Verification items for the finished model (mm, model axes). A direction names the side the tool comes from. Round coordinates to 2 decimals unless told otherwise and drop trailing zeros. Order: outer loops, then holes, each group sorted by start corner. A loop starts at its lowest first (then second) coordinate and runs counter-clockwise, first axis right, second up. Notation, with made-up numbers: M -15.5,8 L 5.5,8 A24 ccw 5.5,31 Z; hole C -9,43 d11. An arc over 180 degrees is marked long. Use one line per item in the form item = value. Start each with the question number.
Item 1: Release check for a two-part mould opening along X. For faces 1 (the flat face through (-39, 5, -6)), 2 (the flat face through (-1, 7, -10)) record: +X half, -X half, draft (parallel to the pull), parting line (faces both ways), or undercut.
Item 2: Cross-section at B-B on x = -41. Enter the section's corners in (y, z), then the cut area to 3 significant figures.
Item 3: Tool access check on faces 3 (the cylindrical face through (-44.173, 1.972, 2.205)), 4 (the flat face through (-21, 4.5, 6)), 5 (the cylindrical face through (-39.61, 6.03, 2.39)). Record the directions out of +Z, -Z, +X, -X, +Y, -Y that give a thin tool (end or side, any length) a straight path to the whole face; none if there is none.
Item 4: Cross-section at C-C on y = 7.25. Enter the section's corners in (x, z), then the cut area to 3 significant figures.
Item 5: Thickness scan on probe 1 along X at (y, z) = (2.5, 1.5); probe 2 along X at (y, z) = (6.25, 4.25); probe 3 along Z at (x, y) = (-31, 7.5). Record the ranges inside material, lowest first. Write a range as [from, to].
Item 6: Cross-section at A-A on z = 6. Enter the section's corners in (x, y), then the cut area to 3 significant figures.
Item 7: Go/stop test with flat-tipped pins: pin 1 Ø5 at (x, z) = (41, 2) entering from -Y; pin 2 Ø1.5 at (x, z) = (-15.5, 4.5) entering from +Y; pin 3 Ø4 at (x, z) = (14, 5) entering from +Y. Record where each tip stops, or that it passes through.
Item 8: Cross-section at D-D on x = 32. Enter the section's corners in (y, z), then the cut area to 3 significant figures.
from build123d import *

# Parameters (mm, degrees)
ESQUISSE1_W             = 90
ESQUISSE1_H             = 25
BOSS_EXTRU_1_DEPTH      = 8
ESQUISSE3_R             = 1.65
ENL_V_MAT_EXTRU_1_DEPTH = 48.384069053
ESQUISSE4_R             = 3.25
ENL_V_MAT_EXTRU_2_DEPTH = 4
EMPREINTE1_START        = -10
EMPREINTE1_DEPTH        = 8
EMPREINTE1_START_2      = 2
EMPREINTE1_2_DEPTH      = 8
EMPREINTE1_START_3      = -38.94589
EMPREINTE1_3_DEPTH      = 77.9
EMPREINTE1_START_4      = -41
EMPREINTE1_4_DEPTH      = 82


with BuildPart() as part:
    # Esquisse1 → Boss.-Extru.1 (new body)
    with BuildSketch(Plane(origin=(0, 0, 0), x_dir=(1, 0, 0), z_dir=(0, 1, 0))):
        Rectangle(ESQUISSE1_W, ESQUISSE1_H)
    extrude(amount=BOSS_EXTRU_1_DEPTH)

    # Esquisse3 → Enlèv. mat.-Extru.1 (cut, through all)
    with BuildSketch(Plane(origin=(0, 8, 0), x_dir=(1, 0, 0), z_dir=(0, 1, 0))):
        with Locations(Location((0, -6, 0), (0, 0, 270))):
            Circle(ESQUISSE3_R)
        with Locations(Location((41, -1.5, 0), (0, 0, 270))):
            Circle(ESQUISSE3_R)
        with Locations(Location((-41, -1.5, 0), (0, 0, 270))):
            Circle(ESQUISSE3_R)
    extrude(amount=-ENL_V_MAT_EXTRU_1_DEPTH, mode=Mode.SUBTRACT)

    # Esquisse4 → Enlèv. mat.-Extru.2 (cut)
    with BuildSketch(Plane.XZ):
        with Locations(Location((-41, 1.5, 0), (0, 0, 270))):
            Circle(ESQUISSE4_R)
        with Locations(Location((41, 1.5, 0), (0, 0, 270))):
            Circle(ESQUISSE4_R)
        with Locations(Location((0, 6, 0), (0, 0, 270))):
            Circle(ESQUISSE4_R)
    extrude(amount=-ENL_V_MAT_EXTRU_2_DEPTH, mode=Mode.SUBTRACT)

    # Empreinte1: read off the stored shape, not the designer's step
    # Empreinte1 outline → Empreinte1 (cut)
    with BuildSketch(Plane.XY.offset(EMPREINTE1_START)):
        Polygon((40, 8), (-40, 8), (-40, 6), (-38.5, 4.5), (38.5, 4.5), (40, 6), align=None)
    extrude(amount=EMPREINTE1_DEPTH, mode=Mode.SUBTRACT)

    # Empreinte1 2 outline → Empreinte1 2 (cut)
    with BuildSketch(Plane.XY.offset(EMPREINTE1_START_2)):
        Polygon((6.5, 4.5), (22.5, 4.5), (24, 6), (24, 8), (5, 8), (5, 6), align=None)
        Polygon((-35.5, 4.5), (-6.5, 4.5), (-5, 6), (-5, 8), (-37, 8), (-37, 6), align=None)
    extrude(amount=EMPREINTE1_2_DEPTH, mode=Mode.SUBTRACT)

    # Empreinte1 3 outline → Empreinte1 3 (add)
    with BuildSketch(Plane.YZ.offset(EMPREINTE1_START_3)):
        Polygon((4.5, 2), (6, 2), (4.5, 3.5), align=None)
        Polygon((4.5, 10), (4.5, 8.5), (6, 10), align=None)
        Polygon((6, -10), (4.5, -8.5), (4.5, -10), align=None)
        Polygon((4.5, -2), (4.5, -3.5), (6, -2), align=None)
    extrude(amount=EMPREINTE1_3_DEPTH)

    # Empreinte1 4 outline → Empreinte1 4 (add)
    with BuildSketch(Plane.YZ.offset(EMPREINTE1_START_4)):
        Polygon((6, -10), (4.5, -8.5), (4.5, -10), align=None)
        Polygon((4.5, -2), (4.5, -3.5), (6, -2), align=None)
    extrude(amount=EMPREINTE1_4_DEPTH)


solid = part.part
Output values:
q1.face_1 = undercut
q1.face_2 = undercut
q2.outline = M 0,-12.5 L 8,-12.5 L 8,-0.15 L 4,-0.15 L 4,-1.75 L 0,-1.75 Z; M 0,4.75 L 4,4.75 L 4,3.15 L 8,3.15 L 8,12.5 L 0,12.5 Z
q2.area = 161 mm2
q3.face_3 = -Y
q3.face_4 = +Y
q3.face_5 = +Y, -Y
q4.outline = M -45,-12.5 L 45,-12.5 L 45,12.5 L -45,12.5 Z; hole C -41,1.5 d3.3; hole M -40,-10 L 40,-10 L 40,-2 L -40,-2 Z; hole M -37,2 L -5,2 L -5,10 L -37,10 Z; hole C 0,6 d3.3; hole M 5,2 L 24,2 L 24,10 L 5,10 Z; hole C 41,1.5 d3.3
q4.area = 1,180 mm2
q5.probe_1 = [-45, -44.25], [-37.75, 37.75], [44.25, 45]
q5.probe_2 = [-45, -37], [-5, 5], [24, 45]
q5.probe_3 = [-12.5, -10], [-2, 2], [10, 12.5]
q6.outline = M -45,0 L -3.25,0 L -3.25,4 L -1.65,4 L -1.65,8 L -5,8 L -5,6 L -6.5,4.5 L -35.5,4.5 L -37,6 L -37,8 L -45,8 Z; M 1.65,4 L 3.25,4 L 3.25,0 L 45,0 L 45,8 L 24,8 L 24,6 L 22.5,4.5 L 6.5,4.5 L 5,6 L 5,8 L 1.65,8 Z
q6.area = 507 mm2
q7.pin_1 = 4
q7.pin_2 = 4.5
q7.pin_3 = 5
q8.outline = M 0,-12.5 L 8,-12.5 L 8,-10 L 6,-10 L 4.5,-8.5 L 4.5,-3.5 L 6,-2 L 8,-2 L 8,12.5 L 0,12.5 Z
q8.area = 174 mm2
